Part print with two shaded views. Sizes in mm from the minimum x, y, z corner. A direction names the side the tool comes from. Give positions to 0.01 mm unless a question says otherwise; leave off trailing zeros. Order: outer loops, then holes, each group sorted by start corner. A loop starts at its lowest first (then second) coordinate and runs counter-clockwise, first axis right, second up. Notation, with made-up numbers: M 28.5,-15 L 63.5,-15 A30 ccw 63.5,7 Z; hole C -20.5,12.5 d4. An arc over 180 degrees is marked long. Return JSON: item names as keys, results as strings.
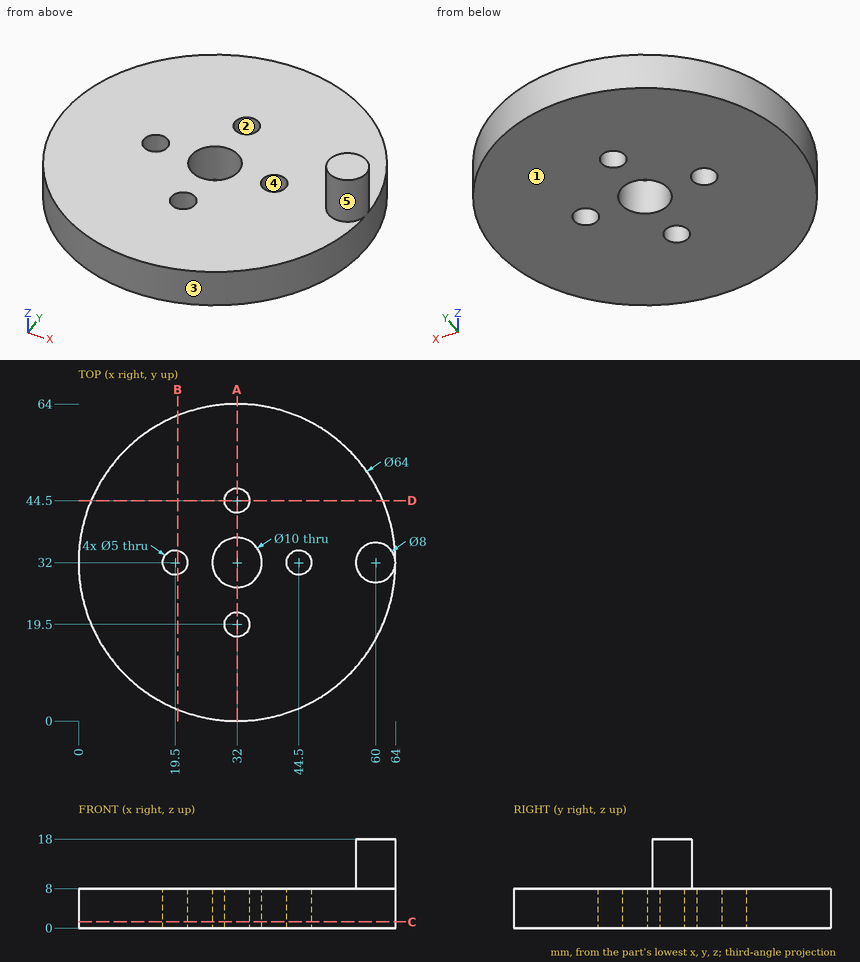
Q1. Two-plate mould, pull along Y, no slides. Class the marked faces 1, 2 and 3: +Y half, -Y half, draft (parallel to the pull), parting line (faces both ways), or undercut.
Established:
{"face 1": "draft", "face 2": "undercut", "face 3": "parting line"}
Q2. Pin check, flat tips, straight feed: pin 1 (10 mm diameter, centred on x = 23.5, z = 11, fed in from +Y); pin 2 (13 mm diameter, centred on x = 32, y = 32, fed in from +Z); pin 3 (6 mm diameter, centred on y = 36, z = 14, fed in from +X). Stop position of each tip, or through.
Established:
{"pin 1": "stops at y = 63.68", "pin 2": "stops at z = 8", "pin 3": "stops at x = 63.87"}
Q3. Band-saw the part on C-C (z = 1.25). Give the cut face in (x, y), then the cut area to 3 significant figures.
Established:
{"outline": "C 32,32 d64; hole C 19.5,32 d5; hole C 32,32 d10; hole C 32,19.5 d5; hole C 32,44.5 d5; hole C 44.5,32 d5", "area": "3,060 mm²"}
Q4. Band-saw the part on A-A (x = 32). Give the cut face in (y, z).
Established:
{"outline": "M 0,0 L 17,0 L 17,8 L 0,8 Z; M 22,0 L 27,0 L 27,8 L 22,8 Z; M 37,0 L 42,0 L 42,8 L 37,8 Z; M 47,0 L 64,0 L 64,8 L 47,8 Z"}
Q5. Band-saw the part on B-B (x = 20). Give the cut face in (y, z), then the cut area to 3 significant figures.
Established:
{"outline": "M 2.34,0 L 29.55,0 L 29.55,8 L 2.34,8 Z; M 34.45,0 L 61.66,0 L 61.66,8 L 34.45,8 Z", "area": "435 mm²"}
Q6. Probe line 1 along Y through (x, z) = (32, 6.25); line 2 along Z through (x, y) = (32, 51.5); line 3 along Y through (x, z) = (43.5, 4). List the from-to ranges inside material, lowest first.
Established:
{"line 1": "y = 0 to 17, 22 to 27, 37 to 42, 47 to 64", "line 2": "z = 0 to 8", "line 3": "y = 2.14 to 29.71, 34.29 to 61.86"}
Q7. Band-saw the part on D-D (y = 44.5). Give the cut face in (x, z).
Established:
{"outline": "M 2.54,0 L 29.5,0 L 29.5,8 L 2.54,8 Z; M 34.5,0 L 61.46,0 L 61.46,8 L 34.5,8 Z"}
Q8. 3-axis set-ups, long thin cutter, end or side, ignore diameter. For the marked faces 4 and 5: which of +Z, -Z, +X, -X, +Y, -Y reach the whole face in a straight line?
Established:
{"face 4": "+Z, -Z", "face 5": "+Z"}
